Source: CAD feature listing. Evaluate the final solid. Frame: model axes, mm. Face numbers are marked on the shaded views. A direction names the side the tool comes from. Coordinates: 2 decimals unless noted, no trailing zeros. Order: outer loops, then holes, each group sorted by start corner. A loop starts at its lowest first (then second) coordinate and runs counter-clockwise, first axis right, second up. Notation, with made-up numbers: (55.25, 7) -> (112.25, 7) arc R19 cw to (112.25, 43) -> close; hole circle Ø4 at (75, -27.5). An arc over 180 degrees is marked (long way). Write item = value, one per line. Start each with the question number.
Item 1: Section query C-C (x = -63.5). Output: boundary loops of the cut face in (y, z).
Item 2: Section query B-B (z = 72). Output: boundary loops of the cut face in (x, y), then the cut area to 3 significant figures.
Item 3: Contact query for flat-ended pins moving along their axis: pin 1 (8 mm diameter, centred on x = 76, z = 87, fed in from +Y); pin 2 (10 mm diameter, centred on y = -52, z = 6, fed in from +X); pin 3 (4 mm diameter, centred on x = 152.5, y = -45.5, fed in from +Z). Output: stop coordinate, or through.
Item 4: Mould query, pull axis Z, two halves, no side actions, for the marked faces 1, 2, 3 and 4. Classes: released by +Z, released by -Z, zero draft, split by the parting line, or undercut.
Item 5: Ray query, line 1 along Y through (x, z) = (192.9, 0); line 2 along X through (y, z) = (-15.5, -25); line 3 along X through (y, z) = (-65.5, -55). Return the intervals inside material, ascending. Write a range as [from, to].
Item 6: Set-up query: the marked faces 5, 6 and 7. Return all of +Z, -Z, +X, -X, +Y, -Y with unobstructed straight access to the full face (end or side cutting, diameter ignored); none if empty.
```python
from build123d import *

# Parameters (mm, degrees)
BOSS_EXTRUDE1_DEPTH = 89
SHELL1_T            = 1
BOSS_EXTRUDE2_DEPTH = 6.5
FILLET1_R           = 2
SKETCH3_R           = 2.9
CUT_EXTRUDE1_DEPTH  = 426.904332073


with BuildPart() as part:
    # Sketch1 → Boss-Extrude1 (new body)
    with BuildSketch(Plane(origin=(0, 0, 0), x_dir=(1, 0, 0), z_dir=(0, 1, 0))):
        with BuildLine():
            Line((-192.5, -37.129148551), (-192.5, -101.5))
            ThreePointArc((-192.5, -101.5), (-182.395183951, -125.895183951), (-158, -136))
            Line((-158, -136), (158, -136))
            ThreePointArc((158, -136), (182.395183951, -125.895183951), (192.5, -101.5))
            Line((192.5, -101.5), (192.5, -37.129148551))
            ThreePointArc((192.5, -37.129148551), (185.5, -25.15), (192.5, -13.170851449))
            Line((192.5, -13.170851449), (192.5, 13.170851449))
            ThreePointArc((192.5, 13.170851449), (185.5, 25.15), (192.5, 37.129148551))
            Line((192.5, 37.129148551), (192.5, 101.5))
            ThreePointArc((192.5, 101.5), (182.395183951, 125.895183951), (158, 136))
            Line((158, 136), (-158, 136))
            ThreePointArc((-158, 136), (-182.395183951, 125.895183951), (-192.5, 101.5))
            Line((-192.5, 101.5), (-192.5, 37.129148551))
            ThreePointArc((-192.5, 37.129148551), (-185.5, 25.15), (-192.5, 13.170851449))
            Line((-192.5, 13.170851449), (-192.5, -13.170851449))
            ThreePointArc((-192.5, -13.170851449), (-185.5, -25.15), (-192.5, -37.129148551))
        make_face()
    extrude(amount=-BOSS_EXTRUDE1_DEPTH)

    # Shell1
    shell1_openings = [part.faces().sort_by_distance(p)[0] for p in [
        (0, 0, 0),
    ]]
    offset(amount=SHELL1_T, openings=shell1_openings, kind=Kind.INTERSECTION)

    # Sketch2 → Boss-Extrude2 (add)
    with BuildSketch(Plane(origin=(0, 0, 0), x_dir=(1, 0, 0), z_dir=(0, 1, 0))):
        with BuildLine():
            Line((-198, -36.833321446), (-198, -101.5))
            ThreePointArc((-198, -101.5), (-186.284271247, -129.784271247), (-158, -141.5))
            Line((-158, -141.5), (158, -141.5))
            ThreePointArc((158, -141.5), (186.284271247, -129.784271247), (198, -101.5))
            Line((198, -101.5), (198, -36.833321446))
            ThreePointArc((198, -36.833321446), (187.5, -25.15), (198, -13.466678554))
            Line((198, -13.466678554), (198, 13.466678554))
            ThreePointArc((198, 13.466678554), (187.5, 25.15), (198, 36.833321446))
            Line((198, 36.833321446), (198, 101.5))
            ThreePointArc((198, 101.5), (186.284271247, 129.784271247), (158, 141.5))
            Line((158, 141.5), (-158, 141.5))
            ThreePointArc((-158, 141.5), (-186.284271247, 129.784271247), (-198, 101.5))
            Line((-198, 101.5), (-198, 36.833321446))
            ThreePointArc((-198, 36.833321446), (-190.510720854, 33.004139036), (-187.5, 25.15))
            ThreePointArc((-187.5, 25.15), (-190.510720854, 17.295860964), (-198, 13.466678554))
            Line((-198, 13.466678554), (-198, -13.466678554))
            ThreePointArc((-198, -13.466678554), (-190.510720854, -17.295860964), (-187.5, -25.15))
            ThreePointArc((-187.5, -25.15), (-190.510720854, -33.004139036), (-198, -36.833321446))
        make_face()
        with BuildLine():
            ThreePointArc((-193.5, 13.770193323), (-186.5, 25.15), (-193.5, 36.529806677))
            Line((-193.5, 36.529806677), (-193.5, 101.5))
            ThreePointArc((-193.5, 101.5), (-183.102290732, 126.602290732), (-158, 137))
            Line((-158, 137), (158, 137))
            ThreePointArc((158, 137), (183.102290732, 126.602290732), (193.5, 101.5))
            Line((193.5, 101.5), (193.5, 36.529806677))
            ThreePointArc((193.5, 36.529806677), (186.5, 25.15), (193.5, 13.770193323))
            Line((193.5, 13.770193323), (193.5, -13.770193323))
            ThreePointArc((193.5, -13.770193323), (186.5, -25.15), (193.5, -36.529806677))
            Line((193.5, -36.529806677), (193.5, -101.5))
            ThreePointArc((193.5, -101.5), (183.102290732, -126.602290732), (158, -137))
            Line((158, -137), (-158, -137))
            ThreePointArc((-158, -137), (-183.102290732, -126.602290732), (-193.5, -101.5))
            Line((-193.5, -101.5), (-193.5, -36.529806677))
            ThreePointArc((-193.5, -36.529806677), (-186.5, -25.15), (-193.5, -13.770193323))
            Line((-193.5, -13.770193323), (-193.5, 13.770193323))
        make_face(mode=Mode.SUBTRACT)
    extrude(amount=-BOSS_EXTRUDE2_DEPTH)

    # Fillet1
    fillet1_edges = [part.edges().sort_by_distance(p)[0] for p in [
        (198, -6.5, 0),
        (198, -6.5, 69.166660723),
        (186.284271247, -6.5, 129.784271247),
        (0, -6.5, 141.5),
        (-186.284271247, -6.5, 129.784271247),
        (-198, 0, 69.166660723),
        (-198, 0, 0),
        (-198, 0, -69.166660723),
        (-186.284271247, -6.5, -129.784271247),
        (0, 0, -141.5),
        (186.284271247, -6.5, -129.784271247),
        (198, -6.5, -69.166660723),
        (-198, -6.5, 69.166660723),
        (-198, -6.5, 0),
        (-198, -6.5, -69.166660723),
        (0, -6.5, -141.5),
        (198, 0, -69.166660723),
        (186.284271247, 0, -129.784271247),
        (-186.284271247, 0, -129.784271247),
        (-186.284271247, 0, 129.784271247),
        (0, 0, 141.5),
        (186.284271247, 0, 129.784271247),
        (198, 0, 69.166660723),
        (198, 0, 0),
        (-182.395183951, 0, 125.895183951),
        (-192.5, 0, 69.314574275),
        (0, 0, 136),
        (182.395183951, 0, 125.895183951),
        (192.5, 0, 69.314574275),
    ]]
    fillet(fillet1_edges, radius=FILLET1_R)

    # Sketch3 → Cut-Extrude1 (cut, through all)
    with BuildSketch(Plane.ZY.offset(193.5)):
        with Locations(Location((0, -47, 0), (0, 0, 180))):
            Circle(SKETCH3_R)
    extrude(amount=-CUT_EXTRUDE1_DEPTH, mode=Mode.SUBTRACT)


solid = part.part
```
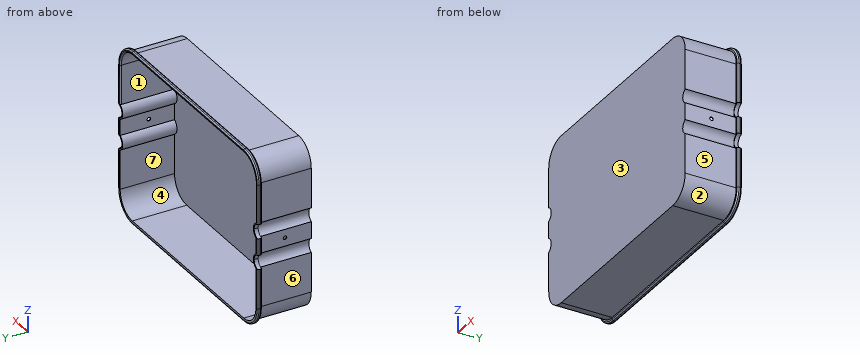
Computed:
q1.outline = (-90, -137) -> (-6.5, -137) -> (-6.5, -139.5) arc R2 ccw to (-4.5, -141.5) -> (-2, -141.5) arc R2 ccw to (0, -139.5) -> (0, -136) -> (-89, -136) -> (-89, 136) -> (-2, 136) arc R2 ccw to (0, 138) -> (0, 139.5) arc R2 ccw to (-2, 141.5) -> (-4.5, 141.5) arc R2 ccw to (-6.5, 139.5) -> (-6.5, 137) -> (-90, 137) -> close
q2.outline = (-198, -4.5) arc R2 ccw to (-196, -6.5) -> (-193.5, -6.5) -> (-193.5, -90) -> (193.5, -90) -> (193.5, -6.5) -> (196, -6.5) arc R2 ccw to (198, -4.5) -> (198, -2) arc R2 ccw to (196, 0) -> (194.5, 0) arc R2 ccw to (192.5, -2) -> (192.5, -89) -> (-192.5, -89) -> (-192.5, -2) arc R2 ccw to (-194.5, 0) -> (-196, 0) arc R2 ccw to (-198, -2) -> close
q2.area = 618 mm^2
q3.pin_1 = -89
q3.pin_2 = 193.5
q3.pin_3 = 137
q4.face_1 = undercut
q4.face_2 = released by -Z
q4.face_3 = zero draft
q4.face_4 = undercut
q5.line_1 = [-90, -49.9], [-44.1, 0]
q5.line_2 = [-186.5, -185.5], [185.5, 186.5]
q5.line_3 = [-193.5, -192.5], [192.5, 193.5]
q6.face_5 = +Z, -Z, +X, -Y
q6.face_6 = +Z, -Z, -X, -Y
q6.face_7 = +Y
